from build123d import *

# Parameters (mm, degrees)
BOSS_EXTRUDE1_DEPTH = 11
CUT_EXTRUDE1_REACH  = 30.128
SKETCH2_R           = 2.25


with BuildPart() as part:
    # Sketch1 → Boss-Extrude1 (new, symmetric)
    with BuildSketch(Plane(origin=(0, 0, 0), x_dir=(1, 0, 0), z_dir=(0, 1, 0))):
        with BuildLine():
            Line((-5.5, -15), (-10.55, -15))
            Line((-10.55, -15), (-10.55, 11.42813746))
            Line((-10.55, 11.42813746), (10.55, 11.42813746))
            Line((10.55, 11.42813746), (10.55, -15))
            Line((10.55, -15), (5.5, -15))
            Line((5.5, -15), (5.5, -5))
            ThreePointArc((5.5, -5), (0, 8.92813746), (-5.5, -5))
            Line((-5.5, -5), (-5.5, -15))
        make_face()
    extrude(amount=BOSS_EXTRUDE1_DEPTH, both=True)

    # Cut-Extrude1: up to this face of the body (flat: up to its plane)
    cut_extrude1_end = Plane(part.part.faces().sort_by_distance((-10.55, 0, 1.78593127))[0])
    # Sketch2 → Cut-Extrude1 (cut, up to the picked face)
    with BuildSketch(Plane(origin=(10.55, 0, 0), x_dir=(0, 0, -1), z_dir=(1, 0, 0)), mode=Mode.PRIVATE) as cut_extrude1_sk1:
        with Locations((-8.5, 0)):
            Circle(SKETCH2_R)
    cut_extrude1_tool1 = split(extrude(cut_extrude1_sk1.sketch, amount=-CUT_EXTRUDE1_REACH, mode=Mode.PRIVATE), bisect_by=cut_extrude1_end, keep=Keep.BOTH, mode=Mode.PRIVATE)
    add(cut_extrude1_tool1.solids().sort_by(Axis((10.55, 0, 8.5), (-1, 0, 0)))[0], mode=Mode.SUBTRACT)


solid = part.part
Check sheet for the modelled part. Datum: model origin and axes. Units: mm. A direction names the side the tool comes from. Give positions to 0.01 mm unless a question says otherwise; leave off trailing zeros. Loops run counter-clockwise (first coordinate to the right, second up) from the corner with the lowest first, then second, coordinate; pieces in that order, holes last. Notation, with made-up numbers: M 64,48 L 123,48 A26 ccw 123,70 Z; hole C 36,5 d3. An arc over 180 degrees is marked long. Answer as a JSON object with one key per item and string values. Group by question number.
Q1. Cross-section at B-B on z = 5.5. Record the cut outline in (x, y).
Q2. Material ranges on line 1 along Y through (x, z) = (8.75, 8.5); line 2 along Z through (x, y) = (0, -2.5); line 3 along Z through (x, y) = (-9, -1), recorded low to high. Write a range as [from, to].
Q3. Release check for a two-part mould opening along X. For faces 1 (the flat face through (7, -11, 5)), 2 (the flat face through (5.5, 0, 11)), 3 (the flat face through (-10.55, 0, 2)) record: released by +X, released by -X, zero draft, split by the parting line, or undercut.
Q4. Cross-section at C-C on z = 8.5. Record the cut outline in (x, y), then the cut area to 3 significant figures.
Q5. Access from +Z, -Z, +X, -X, +Y, -Y to the whole of each face (thin tool, end or side, straight path). Record for faces 4 (the cylindrical face through (8.06, 0.099, 10.748)), 5 (the flat face through (-5.5, 0, 11)).
Q6. Go/stop test with flat-tipped pins: P1, Ø12, axis at x = 1, z = -6.5, coming from the +Y side; P2, Ø2.5, axis at y = 0, z = 8.5, coming from the +X side. Record where each tip stops, or that it passes through.
Q7. Cross-section at D-D on y = -6.5. Record the cut outline in (x, z).
Q8. Cross-section at A-A on y = 0. Record the cut outline in (x, z), then the cut area to 3 significant figures.
Evaluation:
{
 "1": {"outline": "M -10.55,-11 L -5.5,-11 L -5.5,11 L -10.55,11 Z; M 5.5,-11 L 10.55,-11 L 10.55,11 L 5.5,11 Z"},
 "2": {"line 1": "y = [-11, -2.25], [2.25, 11]", "line 2": "z = [-11.43, -8.93]", "line 3": "z = [-11.43, 6.48], [10.52, 15]"},
 "3": {"face 1": "zero draft", "face 2": "undercut", "face 3": "released by -X"},
 "4": {"outline": "M -10.55,-11 L -5.5,-11 L -5.5,-2.25 L -10.55,-2.25 Z; M -10.55,2.25 L -5.5,2.25 L -5.5,11 L -10.55,11 Z; M 5.5,-11 L 10.55,-11 L 10.55,-2.25 L 5.5,-2.25 Z; M 5.5,2.25 L 10.55,2.25 L 10.55,11 L 5.5,11 Z", "area": "177 mm2"},
 "5": {"face 4": "+X, -X", "face 5": "+Z, +Y, -Y"},
 "6": {"P1": "stops at y = 11", "P2": "passes through"},
 "7": {"outline": "M -10.55,-11.43 L 10.55,-11.43 L 10.55,15 L 5.5,15 L 5.5,5 A8.05 cw long -5.5,5 L -5.5,15 L -10.55,15 Z"},
 "8": {"outline": "M -10.55,-11.43 L 10.55,-11.43 L 10.55,6.25 L 5.5,6.25 L 5.5,5 A8.05 cw long -5.5,5 L -5.5,6.25 L -10.55,6.25 Z; M -10.55,10.75 L -5.5,10.75 L -5.5,15 L -10.55,15 Z; M 5.5,10.75 L 10.55,10.75 L 10.55,15 L 5.5,15 Z", "area": "215 mm2"}
}
